Input: part model. Units: mm. Frame: model coordinates. Coordinates: 2 decimals unless noted, no trailing zeros. Loops run counter-clockwise (first coordinate to the right, second up) from the corner with the lowest first, then second, coordinate; pieces in that order, holes last. Notation, with made-up numbers: (-24.75, 60) -> (21.25, 60) arc R9 cw to (21.25, 70) -> close; hole circle Ø1 at (69.25, -28.5). An arc over 180 degrees is marked (long way). Answer as a JSON object with one key per item and string values.
from build123d import *

# Parameters (mm, degrees)
SKETCH_1_W             = 50
SKETCH_1_H             = 19
SKETCH_1_R             = 2
SM_BASE_FLANGE_1_DEPTH = 3
HOLE_WIZARD_M6_1_D     = 5


# Sheet-metal steps are written as plain solids
with BuildPart() as part:
    # Sketch 1 → 基体-法兰1 (new body)
    with BuildSketch(Plane.XY):
        Rectangle(SKETCH_1_W, SKETCH_1_H)
        with Locations((-15, 4)):
            Circle(SKETCH_1_R, mode=Mode.SUBTRACT)
        with Locations(Location((15, 4, 0), (0, 0, 180))):
            Circle(SKETCH_1_R, mode=Mode.SUBTRACT)
    extrude(amount=-SM_BASE_FLANGE_1_DEPTH)

    # M6 螺纹孔1 (through all)
    with Locations(Plane.XY):
        with Locations((0, 4)):
            Hole(HOLE_WIZARD_M6_1_D / 2)


solid = part.part
1. Section query C-C (y = 4). Return loops of the section in (x, z).
Reply:
{"outline": "(-25, -3) -> (-17, -3) -> (-17, 0) -> (-25, 0) -> close; (-13, -3) -> (-2.5, -3) -> (-2.5, 0) -> (-13, 0) -> close; (2.5, -3) -> (13, -3) -> (13, 0) -> (2.5, 0) -> close; (17, -3) -> (25, -3) -> (25, 0) -> (17, 0) -> close"}
2. Section query D-D (x = 15). Return loops of the section in (y, z).
Reply:
{"outline": "(-9.5, -3) -> (2, -3) -> (2, 0) -> (-9.5, 0) -> close; (6, -3) -> (9.5, -3) -> (9.5, 0) -> (6, 0) -> close"}
3. Mould query, pull axis Y, two halves, no side actions, for faces 1 (the face through (0, -9.5, -1)), 2 (the face through (0, 0, 0)), 3 (the face through (16.6, 5.2, -1.5)). Classes: pulls with the +Y half, pulls with the -Y half, needs draft (parallel to the pull), parting line crosses it, or undercut.
Reply:
{"face 1": "pulls with the -Y half", "face 2": "needs draft", "face 3": "undercut"}
4. Section query B-B (x = 0). Return loops of the section in (y, z).
Reply:
{"outline": "(-9.5, -3) -> (1.5, -3) -> (1.5, 0) -> (-9.5, 0) -> close; (6.5, -3) -> (9.5, -3) -> (9.5, 0) -> (6.5, 0) -> close"}
5. Section query A-A (z = -0.5). Return loops of the section in (x, y), plus the area to 3 significant figures.
Reply:
{"outline": "(-25, -9.5) -> (25, -9.5) -> (25, 9.5) -> (-25, 9.5) -> close; hole circle Ø4 at (-15, 4); hole circle Ø5 at (0, 4); hole circle Ø4 at (15, 4)", "area": "905 mm2"}
6. Pin query (flat end, axial travel): P1, Ø5, axis at x = -15, y = 4, coming from the +Z side. Return the tip coordinate at first contact, or that it passes through.
Reply:
{"P1": "stops at z = 0"}
7. Line query: line 1 along Y through (x, z) = (-15, -1.3); line 2 along Y through (x, z) = (0, -2.3); line 3 along X through (y, z) = (5.25, -2.3). Output: solid intervals per line, ascending.
Reply:
{"line 1": "y = -9.5 to 2, 6 to 9.5", "line 2": "y = -9.5 to 1.5, 6.5 to 9.5", "line 3": "x = -25 to -16.56, -13.44 to -2.17, 2.17 to 13.44, 16.56 to 25"}
